Part model, mm, in its own coordinate system. A direction names the side the tool comes from. Coordinates: 2 decimals unless noted, no trailing zeros. Order: outer loops, then holes, each group sorted by start corner. A loop starts at its lowest first (then second) coordinate and runs counter-clockwise, first axis right, second up. Notation, with made-up numbers: M 56.5,62.5 L 96.5,62.5 A25 cw 96.5,74.5 Z; hole C 17,63.5 d2. An arc over 180 degrees is marked long. Answer in a Markdown table with one row per item. Add a question column.
from build123d import *

# Parameters (mm, degrees)
F1_DEPTH = 40
F2_R     = 4
F3_DEPTH = 16


with BuildPart() as f1:
    # F0 (on Front) → F1 (new body)
    with BuildSketch(Plane.XZ):
        with BuildLine():
            Line((19, -29), (19, 29))
            Line((19, 29), (1.5, 29))
            Line((1.5, 29), (1.5, 13.409674))
            ThreePointArc((1.5, 13.409674), (0, -11.5), (-1.5, 13.409674))
            Line((-1.5, 13.409674), (-1.5, 29))
            Line((-1.5, 29), (-19, 29))
            Line((-19, 29), (-19, -29))
            Line((-19, -29), (19, -29))
        make_face()
    extrude(amount=F1_DEPTH)

    # F2 (on face) → F3 (cut)
    with BuildSketch(Plane(origin=(0, 0, -29), x_dir=(1, 0, 0), z_dir=(0, 0, -1))):
        with Locations((-12, 20)):
            Circle(F2_R)
        with Locations((12, 20)):
            Circle(F2_R)
    extrude(amount=-F3_DEPTH, mode=Mode.SUBTRACT)


solid = f1.part
(1) Slice it at B-B (y = -35.5). List the corners of the cut face in (x, z), and give its area (3 significant figures).
(2) Slice it at D-D (z = -23). List the corners of the cut face in (x, y), and give its area (3 significant figures).
(3) Slice it at A-A (z = 1). List the corners of the cut face in (x, y).
(4) Slice it at C-C (x = 4). List the corners of the cut face in (y, z).
(5) 3-axis set-ups, long thin cutter, end or side, ignore diameter. For faces 5 (the flat face through (10, -20, 29)), 6 (the flat face through (12, -20, -13)), 7 (the flat face through (-1.5, -20, 21)): which of +Z, -Z, +X, -X, +Y, -Y reach the whole face in a straight line?
(6) Pull direction X, two halves, no side cores. Call faces 1 (the flat face through (19, -20, 0)), 2 (the cylindrical face through (11.479, -23.966, -21.112)), 3 (the flat face through (0, 0, -12)), 4 (the flat face through (-19, -20, 0)): pulls with the +X half, pulls with the -X half, needs draft (parallel to the pull), parting line crosses it, or undercut.
(7) Wall check: line 1 (Y direction, x = 12, z = -22.25); line 2 (X direction, y = -34.5, z = 1); line 3 (X direction, y = -9, z = -1.5). Give the ranges that are in metal, low to high.
(8) Drop a flat-ended pin along its axis: P1, Ø6.5, axis at x = -12, y = -20, coming from the -Z side. Give the stop position or say it passes through.
Computed:
| question | item | result |
|---|---|---|
| 1 | outline | M -19,-29 L 19,-29 L 19,29 L 1.5,29 L 1.5,13.41 A12.5 cw long -1.5,13.41 L -1.5,29 L -19,29 Z |
| 1 | area | 1,670 mm^2 |
| 2 | outline | M -19,-40 L 19,-40 L 19,0 L -19,0 Z; hole C -12,-20 d8; hole C 12,-20 d8 |
| 2 | area | 1,420 mm^2 |
| 3 | outline | M -19,-40 L -12.5,-40 L -12.5,0 L -19,0 Z; M 12.5,-40 L 19,-40 L 19,0 L 12.5,0 Z |
| 4 | outline | M -40,-29 L 0,-29 L 0,-10.84 L -40,-10.84 Z; M -40,12.84 L 0,12.84 L 0,29 L -40,29 Z |
| 5 | face 5 | +Z, +X, -X, +Y, -Y |
| 5 | face 6 | -Z |
| 5 | face 7 | +Z, +Y, -Y |
| 6 | face 1 | pulls with the +X half |
| 6 | face 2 | undercut |
| 6 | face 3 | needs draft |
| 6 | face 4 | pulls with the -X half |
| 7 | line 1 | y = -40 to -24, -16 to 0 |
| 7 | line 2 | x = -19 to -12.5, 12.5 to 19 |
| 7 | line 3 | x = -19 to -12.25, 12.25 to 19 |
| 8 | P1 | stops at z = -13 |
